```python
from build123d import *

# Parameters (mm, degrees)
SKETCH_1_R          = 11.25
SKETCH_1_R_2        = 2
EXTRUDE_1_DEPTH     = 6
SKETCH_2_R          = 2.55
CUT_EXTRUDE_1_DEPTH = 84.456575535


with BuildPart() as part:
    # Эскиз1 → Бобышка-Вытянуть1 (new body)
    with BuildSketch(Plane(origin=(0, 0, 0), x_dir=(1, 0, 0), z_dir=(0, 1, 0))):
        with BuildLine():
            Line((-32, -24), (-68, -24))
            Line((-68, -24), (-73, -19))
            Line((-73, -19), (-73, 19))
            Line((-73, 19), (-68, 24))
            Line((-68, 24), (-32, 24))
            ThreePointArc((-32, 24), (-27.050252532, 26.050252532), (-25, 31))
            Line((-25, 31), (-25, 34))
            ThreePointArc((-25, 34), (-23.242640687, 38.242640687), (-19, 40))
            Line((-19, 40), (19, 40))
            ThreePointArc((19, 40), (23.242640687, 38.242640687), (25, 34))
            Line((25, 34), (25, -34))
            ThreePointArc((25, -34), (23.242640687, -38.242640687), (19, -40))
            Line((19, -40), (-19, -40))
            ThreePointArc((-19, -40), (-23.242640687, -38.242640687), (-25, -34))
            Line((-25, -34), (-25, -31))
            ThreePointArc((-25, -31), (-27.050252532, -26.050252532), (-32, -24))
        make_face()
        with Locations(Location((-49, 0, 0), (0, 0, 270))):
            Circle(SKETCH_1_R, mode=Mode.SUBTRACT)
        with Locations(Location((-64.5, 15.5, 0), (0, 0, 270))):
            Circle(SKETCH_1_R_2, mode=Mode.SUBTRACT)
        with Locations(Location((-64.5, -15.5, 0), (0, 0, 90))):
            Circle(SKETCH_1_R_2, mode=Mode.SUBTRACT)
        with Locations(Location((-33.5, 15.5, 0), (0, 0, 90))):
            Circle(SKETCH_1_R_2, mode=Mode.SUBTRACT)
        with Locations(Location((-33.5, -15.5, 0), (0, 0, 270))):
            Circle(SKETCH_1_R_2, mode=Mode.SUBTRACT)
    extrude(amount=EXTRUDE_1_DEPTH)

    # Эскиз2 → Вырез-Вытянуть1 (cut, through all)
    with BuildSketch(Plane.XZ):
        with Locations(Location((-17, -30, 0), (0, 0, 270))):
            Circle(SKETCH_2_R)
        with Locations(Location((-17, 30, 0), (0, 0, 90))):
            Circle(SKETCH_2_R)
        with BuildLine():
            Line((16, -32.55), (14, -32.55))
            ThreePointArc((14, -32.55), (11.45, -30), (14, -27.45))
            Line((14, -27.45), (16, -27.45))
            ThreePointArc((16, -27.45), (18.55, -30), (16, -32.55))
        make_face()
        with BuildLine():
            Line((16, 32.55), (14, 32.55))
            ThreePointArc((14, 32.55), (11.45, 30), (14, 27.45))
            Line((14, 27.45), (16, 27.45))
            ThreePointArc((16, 27.45), (18.55, 30), (16, 32.55))
        make_face()
    extrude(amount=-CUT_EXTRUDE_1_DEPTH, mode=Mode.SUBTRACT)


solid = part.part
```
Model file for the job. Use its own axes, mm. A direction names the side the tool comes from. Coordinates: 2 decimals unless noted, no trailing zeros. Order: outer loops, then holes, each group sorted by start corner. A loop starts at its lowest first (then second) coordinate and runs counter-clockwise, first axis right, second up. Notation, with made-up numbers: (74.25, 60) -> (98.25, 60) arc R19 ccw to (98.25, 87) -> close; hole circle Ø1 at (21.25, -21). An arc over 180 degrees is marked (long way). Answer as a JSON object with one key per item and string values. Group by question number.
1) Cut at A-A, the plane y = 4.9. Count the separate pieces of the cut face and the enclosed holes in it, then the cut area to 3 significant figures.
2) Pull direction X, two halves, no side cores. Call faces 4 (the face through (0, 3, 40)), 5 (the face through (23.196, 2.958, -38.289)), 6 (the face through (-25, 3, 33)), 7 (the face through (11.45, 2.96, 30.06)): +X half, -X half, draft (parallel to the pull), parting line (faces both ways), or undercut.
3) Cut at B-B, the plane x = -64.5. Write the cut outline in (y, z).
4) Flat gauge pins, fed straight in: pin 1 (3 mm diameter, centred on x = -49, y = 2.5, fed in from -Z); pin 2 (1.8 mm diameter, centred on x = -46.5, y = 4, fed in from +Z); pin 3 (1.5 mm diameter, centred on y = 3, z = 33, fed in from -X). Where does each tip first touch, or does it go through?
5) Which spindle directions (+Z, -Z, +X, -X, +Y, -Y) get a long thin tool onto all of the face, cutting with end or side? Do faces 1 (the face through (-50, 3, 24)), 2 (the face through (-25, 3, -32)), 3 (the face through (15, 3, 32.55)). Say none if no direction does.
6) Cut at D-D, the plane z = -16. Write the cut outline in (x, y).
7) Cut at C-C, the plane x = -49. Write the cut outline in (y, z), then the cut area to 3 significant figures.
8) Drill centre lines: L1, parallel to X at y = 3.05, z = 15.5; L2, parallel to X at y = 4, z = 0; L3, parallel to X at y = 2.85, z = -30. Where is each one in solid material? Low to high.
Check values:
{
 "1": {"separate pieces": "1", "enclosed holes": "9", "area": "5,720 mm²"},
 "2": {"face 4": "draft", "face 5": "+X half", "face 6": "-X half", "face 7": "undercut"},
 "3": {"outline": "(0, -24) -> (6, -24) -> (6, -17.5) -> (0, -17.5) -> close; (0, -13.5) -> (6, -13.5) -> (6, 13.5) -> (0, 13.5) -> close; (0, 17.5) -> (6, 17.5) -> (6, 24) -> (0, 24) -> close"},
 "4": {"pin 1": "stops at z = -24", "pin 2": "stops at z = 24", "pin 3": "stops at x = -25"},
 "5": {"face 1": "+Z, -X, +Y, -Y", "face 2": "-Z, -X, +Y, -Y", "face 3": "+Y, -Y"},
 "6": {"outline": "(-73, 0) -> (-66.44, 0) -> (-66.44, 6) -> (-73, 6) -> close; (-62.56, 0) -> (-35.44, 0) -> (-35.44, 6) -> (-62.56, 6) -> close; (-31.56, 0) -> (25, 0) -> (25, 6) -> (-31.56, 6) -> close"},
 "7": {"outline": "(0, -24) -> (6, -24) -> (6, -11.25) -> (0, -11.25) -> close; (0, 11.25) -> (6, 11.25) -> (6, 24) -> (0, 24) -> close", "area": "153 mm²"},
 "8": {"L1": "x = -73 to -66.5, -62.5 to -35.5, -31.5 to 25", "L2": "x = -73 to -60.25, -37.75 to 25", "L3": "x = -25.07 to -19.55, -14.45 to 11.45, 18.55 to 25"}
}
